The model under review builds one solid part; all positions refer to its coordinate system, in mm. Coordinates: 2 decimals unless noted, no trailing zeros. Order: outer loops, then holes, each group sorted by start corner. A loop starts at its lowest first (then second) coordinate and runs counter-clockwise, first axis right, second up. Notation, with made-up numbers: (61, -5.5) -> (100, -5.5) arc R5 cw to (100, 2.5) -> close; hole circle Ø10 at (12.25, 0.5). An arc over 180 degrees is marked (long way). Use one line per item in the form item = value.
from build123d import *

# Parameters (mm, degrees)
F0_R     = 10
F1_DEPTH = 25
F2_DEPTH = 50
F3_SIZE  = 3
F4_SIZE  = 3


with BuildPart() as f1:
    # F0 (on Front) → F1 (new body)
    with BuildSketch(Plane.XZ):
        with BuildLine():
            ThreePointArc((2.083333, -24.913043), (18.399502, -16.92508), (25, 0))
            ThreePointArc((25, 0), (18.399502, 16.92508), (2.083333, 24.913043))
            ThreePointArc((2.083333, 24.913043), (-25, 0), (2.083333, -24.913043))
        make_face()
        Circle(F0_R, mode=Mode.SUBTRACT)
        with BuildLine():
            ThreePointArc((2.083333, 24.913043), (18.399502, 16.92508), (25, 0))
            ThreePointArc((25, 0), (18.399502, -16.92508), (2.083333, -24.913043))
            Line((2.083333, -24.913043), (91.458333, -17.43913))
            ThreePointArc((91.458333, -17.43913), (72.5, 0), (91.458333, 17.43913))
            Line((91.458333, 17.43913), (2.083333, 24.913043))
        make_face()
        with BuildLine():
            ThreePointArc((107.5, 0), (102.879651, 11.847556), (91.458333, 17.43913))
            ThreePointArc((91.458333, 17.43913), (72.5, 0), (91.458333, -17.43913))
            ThreePointArc((91.458333, -17.43913), (102.879651, -11.847556), (107.5, 0))
        make_face()
        with Locations((90, 0)):
            Circle(F0_R, mode=Mode.SUBTRACT)
    extrude(amount=F1_DEPTH)

    # F0 (on Front) → F2 (join)
    with BuildSketch(Plane.XZ):
        with BuildLine():
            ThreePointArc((2.083333, -24.913043), (18.399502, -16.92508), (25, 0))
            ThreePointArc((25, 0), (18.399502, 16.92508), (2.083333, 24.913043))
            ThreePointArc((2.083333, 24.913043), (-25, 0), (2.083333, -24.913043))
        make_face()
        Circle(F0_R, mode=Mode.SUBTRACT)
    extrude(amount=F2_DEPTH)

    # F3
    f3_edges = [f1.edges().sort_by_distance(p)[0] for p in [
        (-2.083333, -50, 24.913043),
        (-10, -50, 0),
        (80, -25, 0),
    ]]
    chamfer(f3_edges, length=F3_SIZE)

    # F4
    f4_edges = [f1.edges().sort_by_distance(p)[0] for p in [
        (80, 0, 0),
        (-10, 0, 0),
        (-25, 0, 0),
        (46.770833, 0, -21.176087),
        (46.770833, 0, 21.176087),
        (107.5, 0, 0),
    ]]
    chamfer(f4_edges, length=F4_SIZE)


solid = f1.part
Item 1: Clearance check with flat-ended pins moving along their axes: pin 1 (10 mm diameter, centred on x = 14, y = -5, fed in from +Z); pin 2 (18 mm diameter, centred on x = 90, z = 0, fed in from -Y); pin 3 (3 mm diameter, centred on y = -18.5, z = 0.5, fed in from -X); pin 4 (4 mm diameter, centred on y = -10.5, z = 11, fed in from -X). State where each tip first meets the part, or that it passes through.
Results found:
pin_1 = 24.33
pin_2 = through
pin_3 = -25
pin_4 = -23.32
Item 2: We need section D-D (x = 68.5). Write out the cut boundary in (y, z), plus the area to 3 significant figures.
Results found:
outline = (-25, -19.36) -> (-3, -19.36) -> (0, -16.35) -> (0, 16.35) -> (-3, 19.36) -> (-25, 19.36) -> close
area = 959 mm²
Item 3: We need section A-A (x = 0). Write out the cut boundary in (y, z), plus the area to 3 significant figures.
Results found:
outline = (-50, -22) -> (-47, -25) -> (-3, -25) -> (0, -22) -> (0, -13) -> (-3, -10) -> (-47, -10) -> (-50, -13) -> close; (-50, 13) -> (-47, 10) -> (-3, 10) -> (0, 13) -> (0, 22) -> (-3, 25) -> (-47, 25) -> (-50, 22) -> close
area = 1,460 mm²
Item 4: We need section C-C (z = 2). State how many separate pieces and enclosed holes the cut face has, plus the area to 3 significant figures.
Results found:
separate_pieces = 3
enclosed_holes = 0
area = 3,030 mm²
Item 5: Draft analysis for pull direction Z (two halves, no side actions). For faces 1 (the face through (46.018, -1.479, -19.713)), 2 (the face through (80, -12, 0)), 3 (the face through (9.5, -50, -9.5)), state which applies: released by +Z, released by -Z, zero draft, split by the parting line, or undercut.
Results found:
face_1 = released by -Z
face_2 = undercut
face_3 = zero draft
Item 6: We need section B-B (y = -36.5). Write out the cut boundary in (x, z).
Results found:
outline = (2.08, -24.91) arc R25 ccw to (25, 0) arc R25 ccw to (2.08, 24.91) arc R25 ccw (long way) to start; hole circle Ø20 at (0, 0)
Item 7: To check wall thickness, follow L1, parallel to Z at x = 0, y = -19; L2, parallel to Y at x = 63.5, z = 1; L3, parallel to Z at x = 90, y = -14.25. State the ranges of each line that lie inside material, in increasing order. Write a range as from..to.
Results found:
L1 = -25..-10, 10..25
L2 = -25..0
L3 = -17.56..-10, 10..17.56
